Could you check a few things on this model? Use its own coordinates, in mm. A direction names the side the tool comes from. Round coordinates to 2 decimals unless told otherwise and drop trailing zeros. Order: outer loops, then holes, each group sorted by start corner. A loop starts at its lowest first (then second) coordinate and runs counter-clockwise, first axis right, second up. Notation, with made-up numbers: M -31.75,80.25 L 22.25,80.25 A28 cw 22.25,113.25 Z; hole C -17,0.25 d9. An arc over 180 degrees is marked long. Write each question's results on one line, items separated by ' | '. Start each with the question number.
1. I'm going to push flat-ended pins straight in: pin 1 (1 mm diameter, centred on y = -2, z = 4.5, fed in from +X); pin 2 (1.5 mm diameter, centred on y = -4, z = 5, fed in from -X); pin 3 (1.5 mm diameter, centred on x = 3, y = -3.5, fed in from -Z); pin 4 (0.6 mm diameter, centred on x = 3, y = -2.5, fed in from -Z). Where does each tip first touch, or does it pass through?
2. We'd pull the mould along X, two halves only. Please class faces 1 (the flat face through (2.65, -3.04, 3.39)), 2 (the flat face through (3.86, -3.85, 1.02)), 3 (the flat face through (1.7, -1.7, 9)): released by +X, released by -X, zero draft, split by the parting line, or undercut.
3. Suppose I cut it at A-A on z = 7.25. Write out the boundary of the cut face in (x, y), and give its area (4 significant figures).
4. Suppose I cut it at D-D on x = 2.95. Write out the boundary of the cut face in (y, z), and give its area (3 significant figures).
5. Suppose I cut it at B-B on y = -2.95. Write out the boundary of the cut face in (x, z), and give its area (3 significant figures).
6. Please list where these lines run through material, in increasing order: L1, parallel to Z at x = 3.3, y = -2.95; L2, parallel to Z at x = 3.6, y = -3.5; L3, parallel to X at y = -1.35, z = 7.
7. Suppose I cut it at C-C on z = -0.5. Write out the boundary of the cut face in (x, y), and give its area (3 significant figures).
8. For faces 4 (the flat face through (2.5, -2.5, 5)), 5 (the flat face through (3, -3, 0)), 6 (the flat face through (3.04, -2.65, 3.39)), which set-ups out of +Z, -Z, +X, -X, +Y, -Y let a thin tool reach every point of the face, with its end or its side?
from build123d import *

# Parameters (mm, degrees)
BOX076_W                = 2.9
BOX076_H                = 0.55
BOX076_DEPTH            = 15
BOX077_W                = 1.25
BOX077_H                = 0.55
BOX077_DEPTH            = 6
BOX078_W                = 1.1
BOX078_H                = 0.6
BOX078_DEPTH            = 2
BOX080_W                = 1
BOX080_H                = 0.55
BOX080_DEPTH            = 6
BOX079_W                = 3
BOX079_H                = 0.55
BOX079_DEPTH            = 4
CHAMFER038_SIZE2        = 0.65
CHAMFER038_SIZE         = 2
CHAMFER039_ANGLE        = 33
CHAMFER039_SIZE         = 0.5
CHAMFER041_ANGLE        = 56
CHAMFER041_SIZE         = 0.33
CHAMFER040_ANGLE        = 26.565
CHAMFER040_SIZE         = 1.98
BODY030_PLACEMENT_ANGLE = 135


with BuildPart() as part:
    # Box076 → Box076 (join)
    with BuildSketch(Plane(origin=(-4.95, -0.275, 0), x_dir=(1, 0, 0), z_dir=(0, 0, 1))):
        with Locations((1.45, 0.275)):
            Rectangle(BOX076_W, BOX076_H)
    extrude(amount=BOX076_DEPTH)

    # Box077 → Box077 (cut)
    with BuildSketch(Plane(origin=(-4.125, -0.275, 9), x_dir=(1, 0, 0), z_dir=(0, 0, 1))):
        with Locations((0.625, 0.275)):
            Rectangle(BOX077_W, BOX077_H)
    extrude(amount=BOX077_DEPTH, mode=Mode.SUBTRACT)

    # Box078 → Box078 (cut)
    with BuildSketch(Plane(origin=(-3, -0.3, 13), x_dir=(1, 0, 0), z_dir=(0, 0, 1))):
        with Locations((0.55, 0.3)):
            Rectangle(BOX078_W, BOX078_H)
    extrude(amount=BOX078_DEPTH, mode=Mode.SUBTRACT)

    # Box080 → Box080 (join)
    with BuildSketch(Plane(origin=(-5.95, -0.275, 0), x_dir=(1, 0, 0), z_dir=(0, 0, 1))):
        with Locations((0.5, 0.275)):
            Rectangle(BOX080_W, BOX080_H)
    extrude(amount=BOX080_DEPTH)

    # Box079 → Box079 (cut)
    with BuildSketch(Plane(origin=(-4.95, 0.275, 4), x_dir=(1, 0, 0), z_dir=(0, 0, -1))):
        with Locations((1.5, 0.275)):
            Rectangle(BOX079_W, BOX079_H)
    extrude(amount=BOX079_DEPTH, mode=Mode.SUBTRACT)

    # Chamfer038
    chamfer038_edges = [part.edges().sort_by_distance(p)[0] for p in [
        (-2.05, 0, 4),
    ]]
    chamfer038_side = part.faces().sort_by_distance((-2.05, 0, 8.5))[0]
    chamfer(chamfer038_edges, length=CHAMFER038_SIZE, length2=CHAMFER038_SIZE2, reference=chamfer038_side)

    # Chamfer039
    chamfer039_edges = [part.edges().sort_by_distance(p)[0] for p in [
        (-4.95, 0, 0),
    ]]
    chamfer039_side = part.faces().sort_by_distance((-4.95, 0, 2))[0]
    chamfer(chamfer039_edges, length=CHAMFER039_SIZE, angle=CHAMFER039_ANGLE, reference=chamfer039_side)

    # Chamfer041
    chamfer041_edges = [part.edges().sort_by_distance(p)[0] for p in [
        (-5.95, 0, 0),
    ]]
    chamfer041_side = part.faces().sort_by_distance((-5.612352, 0, 0))[0]
    chamfer(chamfer041_edges, length=CHAMFER041_SIZE, angle=CHAMFER041_ANGLE, reference=chamfer041_side)

    # Chamfer040
    chamfer040_edges = [part.edges().sort_by_distance(p)[0] for p in [
        (-5.95, 0, 6),
    ]]
    chamfer040_side = part.faces().sort_by_distance((-5.95, 0, 3.244623))[0]
    chamfer(chamfer040_edges, length=CHAMFER040_SIZE, angle=CHAMFER040_ANGLE, reference=chamfer040_side)


with BuildPart() as part_1:
    # Body030 placement: moved
    add(part.part.moved(Location((0, 0, -4))).rotate(Axis((0, 0, -4), (0, 0, 1)), BODY030_PLACEMENT_ANGLE))


solid = part_1.part
Filled sheet:
1) pin 1: stops at x = 2.89 | pin 2: stops at x = 2.86 | pin 3: stops at z = -4 | pin 4: stops at z = 0
2) face 1: released by -X | face 2: released by +X | face 3: zero draft
3) outline: M 1.26,-1.64 L 1.84,-2.23 L 2.23,-1.84 L 1.64,-1.26 Z; M 2.72,-3.11 L 3.31,-3.69 L 3.69,-3.31 L 3.11,-2.72 Z | area: 0.9075 mm^2
4) outline: M -3.34,0 L -2.56,0 L -2.56,5 L -2.88,5 L -2.88,11 L -3.34,11 Z | area: 6.62 mm^2
5) outline: M 2.56,0 L 3.34,0 L 3.34,11 L 2.88,11 L 2.88,5 L 2.56,5 Z | area: 6.62 mm^2
6) L1: z = 0 to 11 | L2: z = -3.61 to 1.88 | L3: x = 1.55 to 1.74
7) outline: M 3.31,-3.69 L 4.01,-4.4 L 4.4,-4.01 L 3.69,-3.31 Z | area: 0.550 mm^2
8) face 4: +Z | face 5: -Z, -X, +Y | face 6: +Z, -Z, +X, +Y
